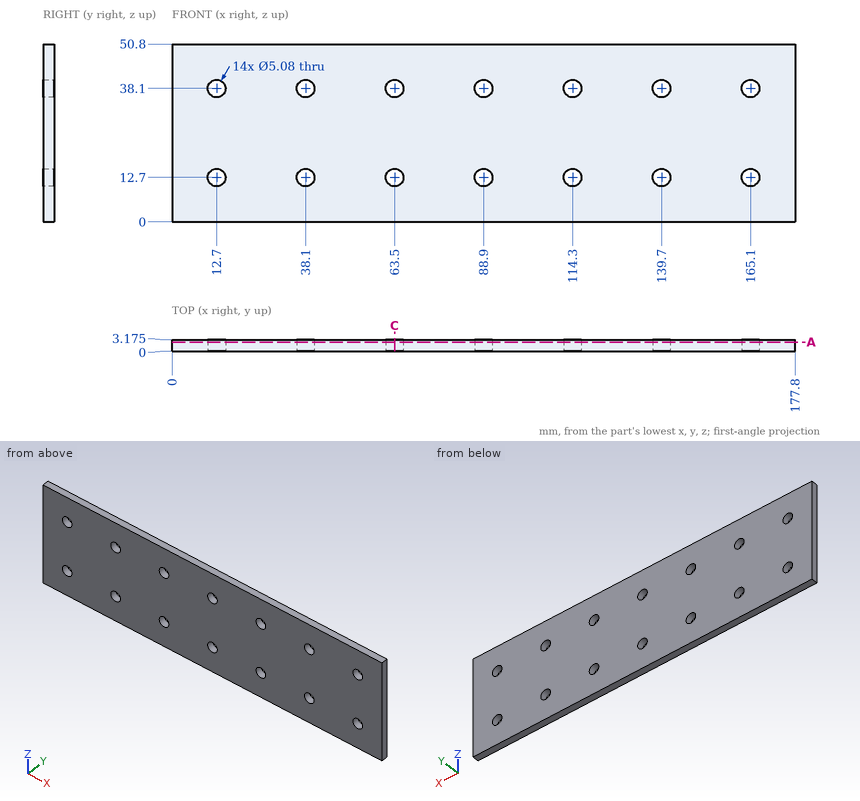
Study the drawing (mm; zero at the part's minimum x, y, z) and answer. Coordinates: 2 decimals unless noted, no trailing zeros. Loops run counter-clockwise (first coordinate to the right, second up) from the corner with the lowest first, then second, coordinate; pieces in that order, holes last. Notation, with made-up numbers: (65.5, -33) -> (117.5, -33) arc R21 ccw to (117.5, -10) -> close; hole circle Ø7 at (4, -14.75). An arc over 180 degrees is marked (long way). Write each question's results on one line, items separated by ' | '. Start each with the question number.
1) A flat-ended cylindrical pin translates along its axis: P1, Ø4.5, axis at x = 139.7, z = 38.1, coming from the +Y side. Find the tip coordinate at first contact, or state that the pin passes through.
2) Find section A-A on y = 2.55. Count the separate pieces of the cut face and the enclosed holes in it, then the cut area to 3 significant figures.
3) Consider line 1 along Z through (x, y) = (139, 2.85). Determine where the line is inside the solid, lowest interval first.
4) Find section C-C on x = 63.5. Determine the outline of the cut face in (y, z) (3 decimals).
Response values:
1) P1: passes through
2) separate pieces: 1 | enclosed holes: 14 | area: 8,750 mm^2
3) line 1: z = 0 to 10.26, 15.14 to 35.66, 40.54 to 50.8
4) outline: (0, 0) -> (3.175, 0) -> (3.175, 10.16) -> (0, 10.16) -> close; (0, 15.24) -> (3.175, 15.24) -> (3.175, 35.56) -> (0, 35.56) -> close; (0, 40.64) -> (3.175, 40.64) -> (3.175, 50.8) -> (0, 50.8) -> close
